Read the model definition and answer for the solid it produces. Units are mm, in the model's axes. A direction names the side the tool comes from. Coordinates: 2 decimals unless noted, no trailing zeros. Write each loop counter-clockwise with the first axis right and the second up, starting at its lowest first coordinate (ties: lowest second). Pieces come first, ordered by that corner, then holes. Notation, with made-up numbers: (-35, 12.5) -> (-17, 12.5) arc R22 cw to (-17, 29.5) -> close; hole circle Ø6 at (23.5, 70). An arc over 180 degrees is marked (long way). Write item = value, one per line. Start each with the question number.
1) Section A-A (x = -13.5) is taken. Determine the outline of the cut face in (y, z).
2) Section C-C (y = -10.5) is taken. Determine the outline of the cut face in (x, z), plus the area to 3 significant figures.
3) A tool of negligible diameter and unlimited length cuts with its end or side. For faces 5 (the face through (10, 1, 1.4)), 6 (the face through (0, -9, -1)), 7 (the face through (-13, 1.6, 0)), 8 (the face through (1, 32.9, 1)), from which of +Z, -Z, +X, -X, +Y, -Y can it reach the whole face along a straight path? Write none if from no direction.
4) For a pull along X with two mould halves and no side action, classify faces 1 (the face through (2.826, 29.928, -5.856)), 2 (the face through (-6.71, 29.93, -0.52)), 3 (the face through (-8.5, 1, 0)), 4 (the face through (13, 1.6, 0)) as released by +X, released by -X, zero draft, split by the parting line, or undercut.
5) Section B-B (y = 15.5) is taken. Determine the outline of the cut face in (x, z), plus the area to 3 significant figures.
6) Find the intervals of material crossed by line 1 along Z through (x, y) = (-16, 1.7); line 2 along Z through (x, y) = (0, -1.5); line 3 along Y through (x, z) = (-3, 2), in increasing order. Write a range as from..to.
7) Flat-ended cylindrical pins translate along their axes: pin 1 Ø2 at (x, z) = (-12, -0.5) entering from -Y; pin 2 Ø6.5 at (x, z) = (0.5, -1) entering from -Y; pin 3 Ø1.8 at (x, z) = (-6, -0.15) entering from +Y; pin 4 Ø2.5 at (x, z) = (6, 0.15) entering from -Y. Find the tip coordinate at first contact, or state that the pin passes through.
from build123d import *

# Parameters (mm, degrees)
ESQUISSE1_R                  = 11
EXTRUSION1_DEPTH             = 31.9
ESQUISSE2_R                  = 3.5
EXTRUSION2_DEPTH             = 1
ESQUISSE3_R                  = 1
EXTRUSION3_DEPTH             = 5.5
CHANFREIN1_SIZE              = 0.25
ESQUISSE4_R                  = 4
EXTRUSION4_DEPTH             = 2.5
ESQUISSE5_R                  = 1
EXTRUSION5_DEPTH             = 13.5
R_P_TITION_CIRCULAIRE1_COUNT = 6
CHANFREIN2_SIZE              = 0.25
ESQUISSE14_W                 = 3.416971917
ESQUISSE14_H                 = 2.8
ENL_V_MAT_EXTRU_5_DEPTH      = 2
R_P_TITION_CIRCULAIRE2_COUNT = 2
ESQUISSE16_W                 = 2.8
ESQUISSE16_H                 = 0.4
EXTRUSION7_DEPTH             = 9.2
ESQUISSE17_W                 = 2.8
ESQUISSE17_H                 = 0.4
EXTRUSION8_DEPTH             = 9.2
CHANFREIN3_SIZE              = 0.7
CHANFREIN4_SIZE              = 0.7
ESQUISSE18_R                 = 0.5
ENL_V_MAT_EXTRU_6_DEPTH      = 37.8
ESQUISSE19_R                 = 0.5
ENL_V_MAT_EXTRU_7_DEPTH      = 37.8


with BuildPart() as part:
    # Esquisse1 → Extrusion1 (new body)
    with BuildSketch(Plane(origin=(0, 0, 0), x_dir=(1, 0, 0), z_dir=(0, 1, 0))):
        Circle(ESQUISSE1_R)
    extrude(amount=EXTRUSION1_DEPTH)

    # Esquisse2 → Extrusion2 (add)
    with BuildSketch(Plane(origin=(0, 31.9, 0), x_dir=(1, 0, 0), z_dir=(0, 1, 0))):
        Circle(ESQUISSE2_R)
    extrude(amount=EXTRUSION2_DEPTH)

    # Esquisse3 → Extrusion3 (add)
    with BuildSketch(Plane(origin=(0, 32.9, 0), x_dir=(1, 0, 0), z_dir=(0, 1, 0))):
        Circle(ESQUISSE3_R)
    extrude(amount=EXTRUSION3_DEPTH)

    # Chanfrein1
    chanfrein1_edges = [part.edges().sort_by_distance(p)[0] for p in [
        (-1, 38.4, 0),
    ]]
    chamfer(chanfrein1_edges, length=CHANFREIN1_SIZE)

    # Esquisse4 → Extrusion4 (add)
    with BuildSketch(Plane.XZ):
        Circle(ESQUISSE4_R)
    extrude(amount=EXTRUSION4_DEPTH)

    # Esquisse5 → Extrusion5 (add)
    with BuildSketch(Plane.XZ.offset(2.5)):
        Circle(ESQUISSE5_R)
    extrude(amount=EXTRUSION5_DEPTH)

    # Esquisse7 → Trou taraudé M2x0.41 (revolve, cut)
    with BuildSketch(Plane(origin=(-2.865237062, 31.9, -5.271661653), x_dir=(0, 0, 1), z_dir=(1, 0, 0))):
        Polygon((0, 0), (0, 4.480688495), (0.8, 4), (0.8, 0), align=None)
    trou_taraud_m2x0_41 = revolve(axis=Axis((-2.865237062, 38.25, -5.271661653), (0, -1, 0)), mode=Mode.SUBTRACT)

    # Répétition circulaire1: Trou taraudé M2x0.41 ×6 about axis
    r_p_tition_circulaire1_axis = Axis((0, 0, 0), (0, 1, 0))
    for i in range(1, R_P_TITION_CIRCULAIRE1_COUNT):
        add(trou_taraud_m2x0_41.rotate(r_p_tition_circulaire1_axis, i * 360 / R_P_TITION_CIRCULAIRE1_COUNT), mode=Mode.SUBTRACT)

    # Chanfrein2
    chanfrein2_edges = [part.edges().sort_by_distance(p)[0] for p in [
        (-1, -16, 0),
    ]]
    chamfer(chanfrein2_edges, length=CHANFREIN2_SIZE)

    # Esquisse14 → Enlèv. mat.-Extru.5 (cut)
    with BuildSketch(Plane.XZ):
        with Locations((-10.208485959, 0)):
            Rectangle(ESQUISSE14_W, ESQUISSE14_H)
    enl_v_mat_extru_5 = extrude(amount=-ENL_V_MAT_EXTRU_5_DEPTH, mode=Mode.SUBTRACT)

    # Répétition circulaire2: Enlèv. mat.-Extru.5 ×2 about axis
    r_p_tition_circulaire2_axis = Axis((0, 0, 0), (0, 1, 0))
    for i in range(1, R_P_TITION_CIRCULAIRE2_COUNT):
        add(enl_v_mat_extru_5.rotate(r_p_tition_circulaire2_axis, i * 360 / R_P_TITION_CIRCULAIRE2_COUNT), mode=Mode.SUBTRACT)

    # Esquisse16 → Extrusion7 (add)
    with BuildSketch(Plane(origin=(8.5, 0, 0), x_dir=(0, 0, -1), z_dir=(1, 0, 0))):
        with Locations((0, 1.8)):
            Rectangle(ESQUISSE16_W, ESQUISSE16_H)
    extrude(amount=EXTRUSION7_DEPTH)

    # Esquisse17 → Extrusion8 (add)
    with BuildSketch(Plane.ZY.offset(8.5)):
        with Locations((0, 1.8)):
            Rectangle(ESQUISSE17_W, ESQUISSE17_H)
    extrude(amount=EXTRUSION8_DEPTH)

    # Chanfrein3
    chanfrein3_edges = [part.edges().sort_by_distance(p)[0] for p in [
        (17.7, 1.8, 1.4),
        (17.7, 1.8, -1.4),
    ]]
    chamfer(chanfrein3_edges, length=CHANFREIN3_SIZE)

    # Chanfrein4
    chanfrein4_edges = [part.edges().sort_by_distance(p)[0] for p in [
        (-17.7, 1.8, -1.4),
        (-17.7, 1.8, 1.4),
    ]]
    chamfer(chanfrein4_edges, length=CHANFREIN4_SIZE)

    # Esquisse18 → Enlèv. mat.-Extru.6 (cut, through all)
    with BuildSketch(Plane.XZ.offset(-1.6)):
        with Locations((-16, 0)):
            Circle(ESQUISSE18_R)
    extrude(amount=-ENL_V_MAT_EXTRU_6_DEPTH, mode=Mode.SUBTRACT)

    # Esquisse19 → Enlèv. mat.-Extru.7 (cut, through all)
    with BuildSketch(Plane.XZ.offset(-1.6)):
        with Locations((16, 0)):
            Circle(ESQUISSE19_R)
    extrude(amount=-ENL_V_MAT_EXTRU_7_DEPTH, mode=Mode.SUBTRACT)


solid = part.part
Answer key:
q1.outline = (1.6, -1.4) -> (2, -1.4) -> (2, 1.4) -> (1.6, 1.4) -> close
q2.outline = circle Ø2 at (0, 0)
q2.area = 3.14 mm^2
q3.face_5 = +X, -Y
q3.face_6 = -Y
q3.face_7 = -X, -Y
q3.face_8 = +Y
q4.face_1 = undercut
q4.face_2 = undercut
q4.face_3 = released by -X
q4.face_4 = zero draft
q5.outline = circle Ø22 at (0, 0)
q5.area = 380 mm^2
q6.line_1 = -1.4..-0.5, 0.5..1.4
q6.line_2 = -4..4
q6.line_3 = -2.5..31.9
q7.pin_1 = 1.6
q7.pin_2 = -16
q7.pin_3 = 31.9
q7.pin_4 = 0
